from build123d import *

# Parameters (mm, degrees)
F0_W     = 1500
F0_H     = 800
F1_DEPTH = 50
F3_DEPTH = 50


with BuildPart() as f1:
    # F0 (on Front) → F1 (new body, symmetric)
    with BuildSketch(Plane.XZ):
        Rectangle(F0_W, F0_H)
    extrude(amount=F1_DEPTH, both=True)

    # F2 (on face) → F3 (join)
    with BuildSketch(Plane(origin=(0, 50, 0), x_dir=(-1, 0, 0), z_dir=(0, 1, 0))):
        Polygon((700, -400), (750, -400), (750, -350), (745, -350), (745, -395), (700, -395), align=None)
        Polygon((-750, -400), (-700, -400), (-700, -395), (-745, -395), (-745, -350), (-750, -350), align=None)
        Polygon((-700, 395), (-700, 400), (-750, 400), (-750, 350), (-745, 350), (-745, 395), align=None)
        Polygon((745, 350), (750, 350), (750, 400), (700, 400), (700, 395), (745, 395), align=None)
    extrude(amount=F3_DEPTH)


solid = f1.part
Could you check a few things on this model? Use its own coordinates, in mm. A direction names the side the tool comes from. Give positions to 0.01 mm unless a question says otherwise; leave off trailing zeros. Order: outer loops, then holes, each group sorted by start corner. A loop starts at its lowest first (then second) coordinate and runs counter-clockwise, first axis right, second up.
Item 1: I need wall thicknesses on line 1 (Y direction, x = -367.5, z = -183). Which ranges of the line are inside material? Lowest first, please.
Item 2: For faces 1 (the face through (-734.1, 100, 395.5)), 2 (the face through (722, 75, -395)), which set-ups out of +Z, -Z, +X, -X, +Y, -Y let a thin tool reach every point of the face, with its end or its side?
Item 3: If we section it at C-C, the plane z = -151: Write out the boundary of the cut face in (x, y), plus the area to 3 significant figures.
Item 4: I'm going to push a flat-ended pin straight in: pin 1 (5 mm diameter, centred on x = -57, z = 34, fed in from +Y). Where does the tip first touch, or does it pass through?
Item 5: If we section it at B-B, the plane x = -331.5: Write out the boundary of the cut face in (y, z), plus the area to 3 significant figures.
Item 6: If we section it at A-A, the plane y = 73.5: Write out the boundary of the cut face in (x, z).
Item 7: If we mould it in two halves opening along X, with no side actions, what happens to faces 3 (the face through (750, 7, -6)), 4 (the face through (-722, 75, 395)), 5 (the face through (10, -9, -400))? For each: pulls with the +X half, pulls with the -X half, needs draft (parallel to the pull), parting line crosses it, or undercut.
Values:
1. line 1: y = -50 to 50
2. face 1: +Z, -Z, +X, -X, +Y
2. face 2: +Y
3. outline: (-750, -50) - (750, -50) - (750, 50) - (-750, 50) - close
3. area: 150,000 mm2
4. pin 1: stops at y = 50
5. outline: (-50, -400) - (50, -400) - (50, 400) - (-50, 400) - close
5. area: 80,000 mm2
6. outline: (-750, -400) - (-700, -400) - (-700, -395) - (-745, -395) - (-745, -350) - (-750, -350) - close; (-750, 350) - (-745, 350) - (-745, 395) - (-700, 395) - (-700, 400) - (-750, 400) - close; (700, -400) - (750, -400) - (750, -350) - (745, -350) - (745, -395) - (700, -395) - close; (700, 395) - (745, 395) - (745, 350) - (750, 350) - (750, 400) - (700, 400) - close
7. face 3: pulls with the +X half
7. face 4: undercut
7. face 5: needs draft
